Autodesk Inventor part; units mm, degrees
ref_plane "YZ Plane" through (0, 0, 0) normal (1, 0, 0) x (0, 1, 0)
ref_plane "XZ Plane" through (0, 0, 0) normal (0, 1, 0) x (-1, 0, 0)
ref_plane "XY Plane" through (0, 0, 0) normal (0, 0, 1) x (1, 0, 0)
sketch "Sketch1" plane through (0, 0, 0) normal (0, 1, 0) x (-1, 0, 0)
  line L0 (33.1724, 3.556) -> (-33.1724, 3.556)
  line L1 (-33.1724, -3.556) -> (33.1724, -3.556)
  line L2 (33.1724, 3.556) -> (-33.1724, -3.556) construction
  line L3 (-33.1724, 3.556) -> (33.1724, -3.556) construction
  arc A0 (33.1724, -3.556) -> (33.1724, 3.556) centre (33.1724, 0) ccw
  arc A1 (-33.1724, 3.556) -> (-33.1724, -3.556) centre (-33.1724, 0) ccw
  circle A2 centre (33.1724, 0) radius 1.3208
  circle A3 centre (-2.3876, 0) radius 1.3208
  circle A4 centre (-33.1724, 0) radius 1.3208
  point P0 (0, 0)
  dimension "d2" = 2.6416
  dimension "d3" = 2.6416
  dimension "d4" = 2.6416
  dimension "d5" = 35.56
extrude "Extrusion1" add sketch "Sketch1" along normal blind 1.016
properties part number "ArmConnector1Mini"
Input: part model. Units: mm. Frame: model coordinates. Coordinates: 2 decimals unless noted, no trailing zeros. Loops run counter-clockwise (first coordinate to the right, second up) from the corner with the lowest first, then second, coordinate; pieces in that order, holes last. Notation, with made-up numbers: M 38,-11 L 53,-11 A28 cw 53,15 Z; hole C 52.25,18.25 d7. An arc over 180 degrees is marked long. One line per item, written item: value.
(1) Line query: line 1 along X through (y, z) = (0.85, 0.5); line 2 along Z through (x, y) = (-33, 0.4); line 3 along X through (y, z) = (0.2, 2.75). Output: solid intervals per line, ascending. Write a range as from..to.
Filled in:
line 1: -36.69..-34.39, -31.95..1.17, 3.61..31.95, 34.39..36.69
line 2: -3.56..-1.31, 1.31..3.56
line 3: -35.43..35.43
(2) Section B-B (y = 0.4). Output: boundary loops of the cut face in (x, z), and give its area (3 significant figures).
Filled in:
outline: M -33.17,-3.56 L 33.17,-3.56 A3.56 ccw 33.17,3.56 L -33.17,3.56 A3.56 ccw Z; hole C -33.17,0 d2.64; hole C 2.39,0 d2.64; hole C 33.17,0 d2.64
area: 495 mm^2
(3) Section A-A (z = 0). Output: boundary loops of the cut face in (x, y).
Filled in:
outline: M -36.73,0 L -34.49,0 L -34.49,1.02 L -36.73,1.02 Z; M -31.85,0 L 1.07,0 L 1.07,1.02 L -31.85,1.02 Z; M 3.71,0 L 31.85,0 L 31.85,1.02 L 3.71,1.02 Z; M 34.49,0 L 36.73,0 L 36.73,1.02 L 34.49,1.02 Z
